For this review, take the finished solid that the model builds, in its own axes (mm). A direction names the side the tool comes from. Round coordinates to 2 decimals unless told otherwise and drop trailing zeros. Order: outer loops, then holes, each group sorted by start corner. A loop starts at its lowest first (then second) coordinate and runs counter-clockwise, first axis right, second up. Notation, with made-up numbers: (-23, 67.5) - (33, 67.5) arc R20 cw to (33, 81.5) - close; hole circle Ø3 at (-25.75, 32). An arc over 180 degrees is marked (long way). Write each question's results on one line, items separated by ' | '. Start each with the question number.
(1) Draft analysis for pull direction Y (two halves, no side actions). For faces 3 (the flat face through (-11, 0, 10.904)), 4 (the flat face through (4, -13.816, 9)), state which applies: pulls with the +Y half, pulls with the -Y half, needs draft (parallel to the pull), parting line crosses it, or undercut.
(2) Take a section at B-B, the plane z = 1.25. Give the boundary of the cut face in (x, y).
(3) Insertion check: pin 1 Ø13 at (x, y) = (7, 3) entering from +Z; pin 2 Ø4 at (y, z) = (-2, 10) entering from -X; pin 3 Ø1 at (x, y) = (-27, -14.5) entering from +Z. Each pin has a flat end and moves straight along its axis. Give the tip position at first contact, or say it passes through.
(4) For faces 1 (the flat face through (6, 0, 8.327)), 2 (the flat face through (1, 1, 0)), list the 3-axis set-ups (+Z, -Z, +X, -X, +Y, -Y) from which the entire face can be reached by the end or side of a thin tool; tool diameter is ignored.
(5) For L1, parallel to Z at x = 1.5, y = 9; L2, parallel to Y at x = -6, z = 2.5; L3, parallel to Z at x = 9, y = -29, list the stretches that pass through material, from the lowest coordinate up. Write a range as from..to.
(6) Take a section at A-A, the plane z = 9.5. Give the boundary of the cut face in (x, y), plus the area to 3 significant figures.
```python
from build123d import *

# Parameters (mm, degrees)
F3_DEPTH      = 37.4664531479
F3_DEPTH_BACK = 37.4664531479
F4_W          = 27.0610069856
F4_H          = 5.9583876282
F5_DEPTH      = 37.4664532479
F6_T1_DEPTH   = 27.0610069856


# Not quite as in the source:
# - a fillet or chamfer that OpenCascade refuses, or shapes differently, is made with other operations: its cross-section is extruded or revolved along the edge and cut away or added


with BuildPart() as f1:
    # F0 (on Front) → F1 (revolve)
    with BuildSketch(Plane.XZ):
        with BuildLine():
            Line((0, 10.9038136992), (0, 0))
            Line((0, 0), (37.4654531479, 0))
            ThreePointArc((37.4654531479, 0), (34.2718000562, 7.7101606075), (26.5616394487, 10.9038136992))
            Line((26.5616394487, 10.9038136992), (0, 10.9038136992))
        make_face()
    revolve(axis=Axis((0, 0, 5.4519068496), (0, 0, 1)))

    # F2 (on Front) → F3 (cut, two sides)
    with BuildSketch(Plane.XZ) as f3_sk:
        Polygon((-10.2507751435, 15.1971811429), (-9.8996739835, 12.9150208086), (41.1855690181, 2.2064307705), (41.1855690181, 15.1971811429), align=None)
    extrude(amount=-F3_DEPTH, mode=Mode.SUBTRACT)
    extrude(f3_sk.sketch, amount=F3_DEPTH_BACK, mode=Mode.SUBTRACT)

    # F4 (on Right) → F5 (cut, through all)
    with BuildSketch(Plane.YZ):
        with Locations((-0.2851500176, 11.3063631579)):
            Rectangle(F4_W, F4_H)
    extrude(amount=F5_DEPTH, mode=Mode.SUBTRACT)

    # F6: fillet of radius 3 on 1 edges, made by hand

    # F6_s2 → F6_t1 (cut)
    with BuildSketch(Plane.XZ.offset(-13.2453534752)):
        with BuildLine():
            ThreePointArc((-2.3845113791, 11.3396775065), (-0.6712164267, 10.2947282416), (0, 8.4034939704))
            Line((0, 8.4034939704), (0, 10.8398314981))
            Line((0, 10.8398314981), (-2.3845113791, 11.3396775065))
        make_face()
    extrude(amount=F6_T1_DEPTH, mode=Mode.SUBTRACT)


solid = f1.part
```
Results below:
1) face 3: needs draft | face 4: undercut
2) outline: circle Ø74.79 at (0, 0)
3) pin 1: stops at z = 8.33 | pin 2: stops at x = -33.91 | pin 3: stops at z = 10.3
4) face 1: +Z, +X | face 2: -Z, +X, -X, +Y, -Y
5) L1: z = 0..8.33 | L2: y = -36.69..36.69 | L3: z = 0..8.95
6) outline: (-0.21, -13.82) - (-0.21, 13.25) - (6.39, 13.25) - (6.39, 31.27) arc R31.91 ccw (long way) to (6.39, -31.27) - (6.39, -13.82) - close | area: 1,830 mm^2
